Here's how the part is built. I have some questions about the finished solid (model axes, mm). A direction names the side the tool comes from. Round coordinates to 2 decimals unless told otherwise and drop trailing zeros. Loops run counter-clockwise (first coordinate to the right, second up) from the corner with the lowest first, then second, coordinate; pieces in that order, holes last. Notation, with made-up numbers: (53.5, -39.5) - (107.5, -39.5) arc R30 cw to (107.5, -13.5) - close; hole circle Ø7 at (8, 58.25). An arc over 180 degrees is marked (long way). Answer as a JSON object with one key per item and string values. Group by question number.
1) Which directions (+Z, -Z, +X, -X, +Y, -Y) give clear straight access to the entire face, cutting with the end or side of a thin tool? Please do faces 1 (the face through (-23, 16, 1)), 2 (the face through (20, -4, 1)).
2) I want a section at B-B, the plane z = 0.6. Please give me the cut outline in (x, y), then the cut area to 3 significant figures.
3) I want a section at C-C, the plane x = -18. Please give me the cut outline in (y, z), then the cut area to 3 significant figures.
4) I want a section at A-A, the plane x = 13. Please give me the cut outline in (y, z).
5) I want a section at D-D, the plane y = -17. Please give me the cut outline in (x, z), then the cut area to 3 significant figures.
6) If I drill on line 1 along Y through (x, z) = (-12.5, 1.85); line 2 along X through (y, z) = (28, 0.45); line 3 along X through (y, z) = (-8, 0.7), over which ranges is the centre line in solid material (lowest first)? Write a range as [from, to].
7) If we mould it in two halves opening along X, with no side actions, what happens to faces 3 (the face through (23, 16, 1)), 4 (the face through (-20, -4, 1)), 5 (the face through (-17, -20, 1))? For each: pulls with the +X half, pulls with the -X half, needs draft (parallel to the pull), parting line crosses it, or undercut.
8) Will this pin go through, and if not, where does the flat tip stop? P1, Ø1, axis at y = -23, z = 1, coming from the -X side.
from build123d import *

# Parameters (mm, degrees)
BOSS_EXTRUDE1_DEPTH = 2


with BuildPart() as part:
    # Sketch1 → Boss-Extrude1 (new body)
    with BuildSketch(Plane.XY):
        with BuildLine():
            Line((-13, 17), (-13, -4))
            Line((-13, -4), (17, -4))
            Line((17, -4), (17, 17.937742252))
            ThreePointArc((17, 17.937742252), (8.654858798, 18.118391793), (4.047290897, 25.078588197))
            Line((4.047290897, 25.078588197), (-4.047290897, 25.078588197))
            ThreePointArc((-4.047290897, 25.078588197), (-6.970601449, 19.318207343), (-13, 17))
        make_face()
        with BuildLine():
            Line((-23, 0), (-23, -4))
            Line((-23, -4), (-17, -4))
            Line((-17, -4), (-17, 17.937742252))
            ThreePointArc((-17, 17.937742252), (-22, 26), (-17, 34.062257748))
            Line((-17, 34.062257748), (-17, 36))
            Line((-17, 36), (-23, 36))
            Line((-23, 36), (-23, 0))
        make_face()
        with BuildLine():
            Line((17, 36), (-17, 36))
            Line((-17, 36), (-17, 34.062257748))
            ThreePointArc((-17, 34.062257748), (-8.25658351, 33.64852927), (-4, 26))
            ThreePointArc((-4, 26), (-4.0118305, 25.538687704), (-4.047290897, 25.078588197))
            Line((-4.047290897, 25.078588197), (4.047290897, 25.078588197))
            ThreePointArc((4.047290897, 25.078588197), (7.870778664, 33.395342351), (17, 34.062257748))
            Line((17, 34.062257748), (17, 36))
        make_face()
        with BuildLine():
            Line((17, 17.937742252), (17, -4))
            Line((17, -4), (23, -4))
            Line((23, -4), (23, 0))
            Line((23, 0), (23, 36))
            Line((23, 36), (17, 36))
            Line((17, 36), (17, 34.062257748))
            ThreePointArc((17, 34.062257748), (20.64852927, 30.74341649), (22, 26))
            ThreePointArc((22, 26), (20.64852927, 21.25658351), (17, 17.937742252))
        make_face()
        Polygon((-13, -4), (-17, -4), (-17, -36), (17, -36), (17, -4), align=None)
        with BuildLine():
            Line((-17, 17.937742252), (-17, -4))
            Line((-17, -4), (-13, -4))
            Line((-13, -4), (-13, 17))
            ThreePointArc((-13, 17), (-15.054224947, 17.237571121), (-17, 17.937742252))
        make_face()
    extrude(amount=BOSS_EXTRUDE1_DEPTH)


solid = part.part
Outcome:
{
 "1": {"face 1": "+Z, -Z, -X, +Y, -Y", "face 2": "+Z, -Z, +X, -Y"},
 "2": {"outline": "(-23, -4) - (-17, -4) - (-17, -36) - (17, -36) - (17, -4) - (23, -4) - (23, 36) - (-23, 36) - close; hole circle Ø18 at (-13, 26); hole circle Ø18 at (13, 26)", "area": "2,420 mm^2"},
 "3": {"outline": "(-4, 0) - (18.52, 0) - (18.52, 2) - (-4, 2) - close; (33.48, 0) - (36, 0) - (36, 2) - (33.48, 2) - close", "area": "50.1 mm^2"},
 "4": {"outline": "(-36, 0) - (17, 0) - (17, 2) - (-36, 2) - close; (35, 0) - (36, 0) - (36, 2) - (35, 2) - close"},
 "5": {"outline": "(-17, 0) - (17, 0) - (17, 2) - (-17, 2) - close", "area": "68.0 mm^2"},
 "6": {"line 1": "[-36, 17.01], [34.99, 36]", "line 2": "[-23, -21.77], [-4.23, 4.23], [21.77, 23]", "line 3": "[-17, 17]"},
 "7": {"face 3": "pulls with the +X half", "face 4": "needs draft", "face 5": "pulls with the -X half"},
 "8": {"P1": "x = -17"}
}
